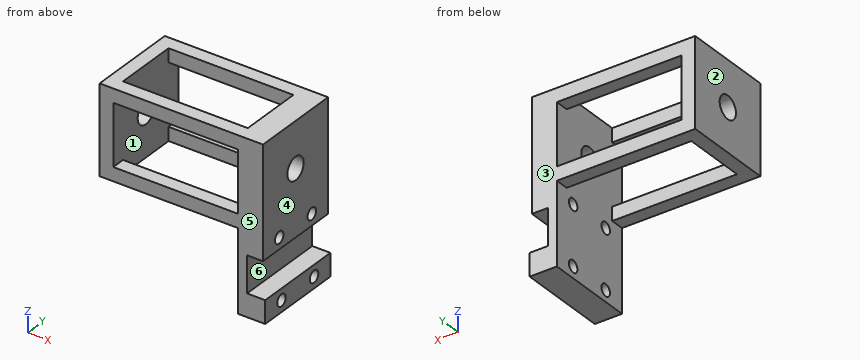
```python
from build123d import *

# Parameters (mm, degrees)
BOSS_EXTRUDE1_DEPTH = 20
SKETCH4_W           = 30.5
SKETCH4_H           = 19.5
BOSS_EXTRUDE2_DEPTH = 20
CUT_EXTRUDE1_REACH  = 51.015
SKETCH6_W           = 27.5
SKETCH6_H           = 13.5
SKETCH7_W           = 27.5
SKETCH7_H           = 14
CUT_EXTRUDE2_DEPTH  = 58.610327885
SKETCH9_R           = 2.5
CUT_EXTRUDE3_DEPTH  = 48.138494794
CUT_EXTRUDE4_REACH  = 49.138
SKETCH10_R          = 1.3
CUT_EXTRUDE5_REACH  = 48.752
SKETCH11_R          = 1.3


with BuildPart() as part:
    # Sketch1 → Boss-Extrude1 (new body)
    with BuildSketch(Plane(origin=(0, 0, 0), x_dir=(-1, 0, 0), z_dir=(0, 1, 0))):
        Polygon((2.893442623, -2.368852459), (2.893442623, 22.131147541), (8.393442623, 22.131147541), (8.393442623, -15.368852459), (2.393442623, -15.368852459), (2.393442623, -10.368852459), (6.393442623, -10.368852459), (6.393442623, -2.368852459), align=None)
    extrude(amount=BOSS_EXTRUDE1_DEPTH)

    # Sketch4 → Boss-Extrude2 (add)
    with BuildSketch(Plane(origin=(0, 20, 0), x_dir=(-1, 0, 0), z_dir=(0, 1, 0))):
        with Locations((23.643442623, 12.381147541)):
            Rectangle(SKETCH4_W, SKETCH4_H)
    extrude(amount=-BOSS_EXTRUDE2_DEPTH)

    # Sketch6 → Cut-Extrude1 (cut, up to next)
    with BuildSketch(Plane(origin=(0, 20, 0), x_dir=(-1, 0, 0), z_dir=(0, 1, 0)), mode=Mode.PRIVATE) as cut_extrude1_sk1:
        with Locations((22.143442623, 12.381147541)):
            Rectangle(SKETCH6_W, SKETCH6_H)
    cut_extrude1_tool1 = extrude(cut_extrude1_sk1.sketch, amount=-CUT_EXTRUDE1_REACH, mode=Mode.PRIVATE) & part.part
    add(cut_extrude1_tool1.solids().sort_by_distance((-22.143443, 20, 12.381148))[0], mode=Mode.SUBTRACT)

    # Sketch7 → Cut-Extrude2 (cut, through all)
    with BuildSketch(Plane.XY.offset(22.131147541)):
        with Locations((-22.143442623, 10)):
            Rectangle(SKETCH7_W, SKETCH7_H)
    extrude(amount=-CUT_EXTRUDE2_DEPTH, mode=Mode.SUBTRACT)

    # Sketch9 → Cut-Extrude3 (cut, through all)
    with BuildSketch(Plane(origin=(-38.893442623, 0, 0), x_dir=(0, -1, 0), z_dir=(-1, 0, 0))):
        with Locations(Location((-10, 12.131147541, 0), (0, 0, 90))):
            Circle(SKETCH9_R)
    extrude(amount=-CUT_EXTRUDE3_DEPTH, mode=Mode.SUBTRACT)

    # Sketch10 → Cut-Extrude4 (cut, up to next)
    with BuildSketch(Plane.YZ.offset(-2.393442623), mode=Mode.PRIVATE) as cut_extrude4_sk1:
        with Locations(Location((5, -12.868852459, 0), (0, 0, 270))):
            Circle(SKETCH10_R)
    cut_extrude4_tool1 = extrude(cut_extrude4_sk1.sketch, amount=-CUT_EXTRUDE4_REACH, mode=Mode.PRIVATE) & part.part
    # Sketch10 → Cut-Extrude4 (cut, up to next)
    with BuildSketch(Plane.YZ.offset(-2.393442623), mode=Mode.PRIVATE) as cut_extrude4_sk2:
        with Locations(Location((15, -12.868852459, 0), (0, 0, 270))):
            Circle(SKETCH10_R)
    cut_extrude4_tool2 = extrude(cut_extrude4_sk2.sketch, amount=-CUT_EXTRUDE4_REACH, mode=Mode.PRIVATE) & part.part
    add(cut_extrude4_tool1.solids().sort_by_distance((-2.393443, 5, -12.868852))[0], mode=Mode.SUBTRACT)
    add(cut_extrude4_tool2.solids().sort_by_distance((-2.393443, 15, -12.868852))[0], mode=Mode.SUBTRACT)

    # Sketch11 → Cut-Extrude5 (cut, up to next)
    with BuildSketch(Plane.YZ.offset(-2.893442623), mode=Mode.PRIVATE) as cut_extrude5_sk1:
        with Locations(Location((5, 0.131147541, 0), (0, 0, 270))):
            Circle(SKETCH11_R)
    cut_extrude5_tool1 = extrude(cut_extrude5_sk1.sketch, amount=-CUT_EXTRUDE5_REACH, mode=Mode.PRIVATE) & part.part
    # Sketch11 → Cut-Extrude5 (cut, up to next)
    with BuildSketch(Plane.YZ.offset(-2.893442623), mode=Mode.PRIVATE) as cut_extrude5_sk2:
        with Locations(Location((15, 0.131147541, 0), (0, 0, 270))):
            Circle(SKETCH11_R)
    cut_extrude5_tool2 = extrude(cut_extrude5_sk2.sketch, amount=-CUT_EXTRUDE5_REACH, mode=Mode.PRIVATE) & part.part
    add(cut_extrude5_tool1.solids().sort_by_distance((-2.893443, 5, 0.131148))[0], mode=Mode.SUBTRACT)
    add(cut_extrude5_tool2.solids().sort_by_distance((-2.893443, 15, 0.131148))[0], mode=Mode.SUBTRACT)


solid = part.part
```
Here's how the part is built. I have some questions about the finished solid (model axes, mm). Face numbers are marked on the shaded views. A direction names the side the tool comes from. Give positions to 0.01 mm unless a question says otherwise; leave off trailing zeros. Loops run counter-clockwise (first coordinate to the right, second up) from the corner with the lowest first, then second, coordinate; pieces in that order, holes last. Notation, with made-up numbers: M 41.5,-22 L 45.5,-22 A22 cw 45.5,-9 Z; hole C -5.75,5 d7. An arc over 180 degrees is marked long. Return JSON: item names as keys, results as strings.
Item 1: Imagine slicing it at C-C on x = -32. List the corners of the cut face in (y, z) for me.
A:
{"outline": "M 0,2.63 L 3,2.63 L 3,5.63 L 0,5.63 Z; M 0,19.13 L 3,19.13 L 3,22.13 L 0,22.13 Z; M 17,2.63 L 20,2.63 L 20,5.63 L 17,5.63 Z; M 17,19.13 L 20,19.13 L 20,22.13 L 17,22.13 Z"}
Item 2: On a 3-axis mill with a long thin cutter (end or side, diameter ignored), from which of +Z, -Z, +X, -X, +Y, -Y can I reach the whole of each face in a straight line? I mean the marked faces 4, 5 and 6. Say none if no direction works.
A:
{"face 4": "+Z, +X, +Y, -Y", "face 5": "+Z, -Z, +X, -X, -Y", "face 6": "+X, +Y, -Y"}
Item 3: Imagine slicing it at A-A on z = 7. List the corners of the cut face in (x, y) for me.
A:
{"outline": "M -38.89,0 L -35.89,0 L -35.89,20 L -38.89,20 Z; M -8.39,0 L -2.89,0 L -2.89,20 L -8.39,20 Z"}
Item 4: Imagine slicing it at D-D on y = 9.5. List the corners of the cut face in (x, z) for me.
A:
{"outline": "M -38.89,2.63 L -35.89,2.63 L -35.89,9.68 L -38.89,9.68 Z; M -38.89,14.58 L -35.89,14.58 L -35.89,22.13 L -38.89,22.13 Z; M -8.39,-15.37 L -2.39,-15.37 L -2.39,-10.37 L -6.39,-10.37 L -6.39,-2.37 L -2.89,-2.37 L -2.89,9.68 L -8.39,9.68 Z; M -8.39,14.58 L -2.89,14.58 L -2.89,22.13 L -8.39,22.13 Z"}
Item 5: I'm going to push flat-ended pins straight in: pin 1 Ø3 at (x, y) = (-10.5, 10) entering from -Z; pin 2 Ø3.5 at (y, z) = (5, 0.13) entering from +X; pin 3 Ø0.9 at (x, y) = (-26, 19) entering from -Z. Where does each tip first touch, or does it pass through?
A:
{"pin 1": "passes through", "pin 2": "stops at x = -2.89", "pin 3": "stops at z = 2.63"}
Item 6: Thinking about a two-plate mould opening in Y: for the marked faces 1, 2 and 3, which applies, released by +Y, released by -Y, zero draft, split by the parting line, or undercut?
A:
{"face 1": "undercut", "face 2": "zero draft", "face 3": "released by +Y"}
Item 7: Please list where these lines run through material, in increasing order: line 1 (X direction, y = 11.75, z = 20); line 2 (Z direction, x = -9.5, y = 1.5); line 3 (X direction, y = 13.75, z = -7).
A:
{"line 1": "x = -38.89 to -35.89, -8.39 to -2.89", "line 2": "z = 2.63 to 5.63, 19.13 to 22.13", "line 3": "x = -8.39 to -6.39"}
Item 8: Imagine slicing it at B-B on y = 1.5. List the corners of the cut face in (x, z) for me, then the cut area to 3 significant figures.
A:
{"outline": "M -38.89,2.63 L -8.39,2.63 L -8.39,-15.37 L -2.39,-15.37 L -2.39,-10.37 L -6.39,-10.37 L -6.39,-2.37 L -2.89,-2.37 L -2.89,22.13 L -38.89,22.13 Z; hole M -35.89,5.63 L -8.39,5.63 L -8.39,19.13 L -35.89,19.13 Z", "area": "404 mm^2"}
